Autodesk Inventor part; units mm, degrees
ref_plane "YZ Plane" through (0, 0, 0) normal (1, 0, 0) x (0, 1, 0)
ref_plane "XZ Plane" through (0, 0, 0) normal (0, 1, 0) x (-1, 0, 0)
ref_plane "XY Plane" through (0, 0, 0) normal (0, 0, 1) x (1, 0, 0)
sketch "Sketch1" plane through (0, 0, 0) normal (0, 0, 1) x (1, 0, 0)
  line L0 (0, 0) -> (25, 0)
  line L1 (25, 0) -> (25, 10)
  line L2 (25, 10) -> (0, 10)
  line L3 (0, 10) -> (0, 0)
  dimension "d0" = 25
  dimension "d1" = 10
extrude "Extrusion1" add sketch "Sketch1" along normal blind 1
sketch "Sketch2" plane through (0, 0, 1) normal (0, 0, 1) x (1, 0, 0)
  circle A0 centre (12.5, 5) radius 1.45
  line L0 (0, 0) -> (25, 0)
  line L1 (0, 10) -> (0, 0)
  line L2 (12.5, 0) -> (12.5, 2.5918) construction
  line L3 (25, 0) -> (25, 10)
  line L4 (25, 10) -> (0, 10)
  line L5 (25, 5) -> (1.9186, 5) construction
  dimension "d4" = 2.9
extrude "Extrusion2" cut sketch "Sketch2" against normal blind 15 contours A0
sketch "Sketch3" plane through (0, 0, 1) normal (0, 0, 1) x (1, 0, 0)
  line L0 (25, 0) -> (25, 10)
  line L1 (0, 10) -> (0, 0)
  circle A0 centre (23.5, 5) radius 0.1
  circle A1 centre (1.5, 5) radius 0.1
  line L2 (25, 5) -> (0, 5) construction
  dimension "d7" = 0.2
  dimension "d8" = 0.2
  dimension "d9" = 1.5
  dimension "d10" = 1.5
extrude "Extrusion3" cut sketch "Sketch3" against normal blind 15
properties part number "MaterialTest01"
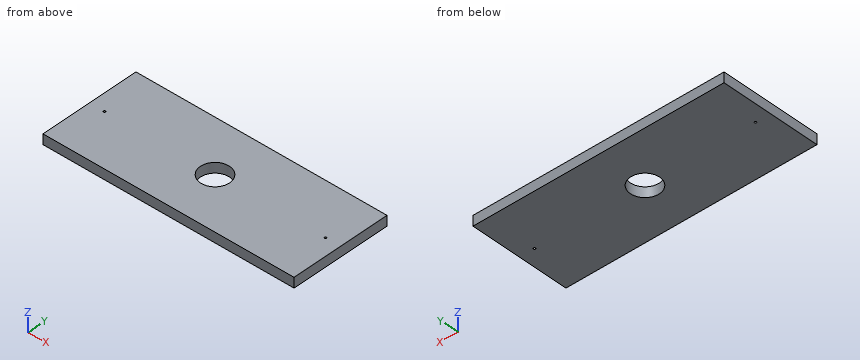
Verification items for the finished model (mm, model axes). Round coordinates to 2 decimals unless told otherwise and drop trailing zeros. Loops run counter-clockwise (first coordinate to the right, second up) from the corner with the lowest first, then second, coordinate; pieces in that order, holes last. Notation, with made-up numbers: (18, 0) - (31, 0) arc R28 cw to (31, 32) - close; hole circle Ø1 at (-6.5, -38.75). An arc over 180 degrees is marked (long way). Answer in a Markdown table with one row per item. Add a question column.
Q1. Material ranges on line 1 (Y direction, x = 12.5, z = 0.25); line 2 (Y direction, x = 1.5, z = 0.65); line 3 (X direction, y = 5.75, z = 0.95), recorded low to high.
Q2. Section check A-A on z = 0.8. Enter the section's corners in (x, y), plus the area to 3 significant figures.
Q3. Section check B-B on x = 12.5. Enter the section's corners in (y, z).
Found:
| question | item | result |
|---|---|---|
| 1 | line 1 | y = 0 to 3.55, 6.45 to 10 |
| 1 | line 2 | y = 0 to 4.9, 5.1 to 10 |
| 1 | line 3 | x = 0 to 11.26, 13.74 to 25 |
| 2 | outline | (0, 0) - (25, 0) - (25, 10) - (0, 10) - close; hole circle Ø0.2 at (1.5, 5); hole circle Ø2.9 at (12.5, 5); hole circle Ø0.2 at (23.5, 5) |
| 2 | area | 243 mm² |
| 3 | outline | (0, 0) - (3.55, 0) - (3.55, 1) - (0, 1) - close; (6.45, 0) - (10, 0) - (10, 1) - (6.45, 1) - close |
